Could you check a few things on this model? Use its own coordinates, in mm. A direction names the side the tool comes from. Round coordinates to 2 decimals unless told otherwise and drop trailing zeros. Write each loop counter-clockwise with the first axis right and the second up, starting at its lowest first coordinate (ties: lowest second). Pieces come first, ordered by that corner, then holes. Notation, with made-up numbers: (20.5, -37.5) -> (77.5, -37.5) arc R7 ccw to (77.5, -29.5) -> close; hole circle Ø11 at (40, -31.75). An arc over 180 degrees is marked (long way). Answer in a Markdown table with one row per item.
from build123d import *

# Parameters (mm, degrees)
SKETCH1_W           = 26
SKETCH1_H           = 10.8
BOSS_EXTRUDE1_DEPTH = 25
SKETCH2_W           = 8
SKETCH2_H           = 4
BOSS_EXTRUDE2_DEPTH = 10.25
SKETCH3_R           = 1.25
CUT_EXTRUDE1_DEPTH  = 10.25
CUT_EXTRUDE2_DEPTH  = 40.092230686
SHELL1_START        = -2.4
SHELL1_DEPTH        = 4.8
SKETCH5_W           = 4.8
SKETCH5_H           = 4.8
CUT_EXTRUDE3_DEPTH  = 10.25
SKETCH6_W           = 1
SKETCH6_H           = 1
CUT_EXTRUDE4_DEPTH  = 45.133009188
SKETCH7_W           = 1
SKETCH7_H           = 1
CUT_EXTRUDE5_DEPTH  = 10.25
FILLET1_R           = 2
FILLET2_R           = 2


# Read off the part's stored shape, not the designer's step: Shell1
with BuildPart() as part:
    # Sketch1 → Boss-Extrude1 (new body)
    with BuildSketch(Plane(origin=(0, 0, 0), x_dir=(1, 0, 0), z_dir=(0, 1, 0))):
        Rectangle(SKETCH1_W, SKETCH1_H)
    extrude(amount=BOSS_EXTRUDE1_DEPTH)

    # Sketch2 → Boss-Extrude2 (add)
    with BuildSketch(Plane(origin=(0, 25, 0), x_dir=(1, 0, 0), z_dir=(0, 1, 0))):
        with Locations((9, 0)):
            Rectangle(SKETCH2_W, SKETCH2_H)
    extrude(amount=BOSS_EXTRUDE2_DEPTH)

    # Sketch3 → Cut-Extrude1 (cut)
    with BuildSketch(Plane.XY.offset(2)):
        with Locations((9, 31.25)):
            Circle(SKETCH3_R)
        with BuildLine():
            Line((5, 31.25), (5, 37.25))
            Line((5, 37.25), (13, 37.25))
            Line((13, 37.25), (13, 31.25))
            ThreePointArc((13, 31.25), (9, 35.25), (5, 31.25))
        make_face()
    extrude(amount=-CUT_EXTRUDE1_DEPTH, mode=Mode.SUBTRACT)

    # Sketch4 → Cut-Extrude2 (cut, through all)
    with BuildSketch(Plane.XY.offset(5.4)):
        Polygon((-13, 0), (-2.8, 25), (-13, 25), align=None)
    extrude(amount=-CUT_EXTRUDE2_DEPTH, mode=Mode.SUBTRACT)

    # Shell1 outline → Shell1 (cut)
    with BuildSketch(Plane.XY.offset(SHELL1_START)):
        Polygon((10, 0), (10, 22), (-0.783911112, 22), (-9.759911112, 0), align=None)
    extrude(amount=SHELL1_DEPTH, mode=Mode.SUBTRACT)

    # Sketch5 → Cut-Extrude3 (cut)
    with BuildSketch(Plane(origin=(0, 25, 0), x_dir=(1, 0, 0), z_dir=(0, 1, 0))):
        with Locations((1.65, 0)):
            Rectangle(SKETCH5_W, SKETCH5_H)
    extrude(amount=-CUT_EXTRUDE3_DEPTH, mode=Mode.SUBTRACT)

    # Sketch6 → Cut-Extrude4 (cut, through all)
    with BuildSketch(Plane(origin=(13, 0, 0), x_dir=(0, 0, -1), z_dir=(1, 0, 0))):
        with Locations((-4.9, 0.5)):
            Rectangle(SKETCH6_W, SKETCH6_H)
        with Locations((4.9, 0.5)):
            Rectangle(SKETCH6_W, SKETCH6_H)
    extrude(amount=-CUT_EXTRUDE4_DEPTH, mode=Mode.SUBTRACT)

    # Sketch7 → Cut-Extrude5 (cut)
    with BuildSketch(Plane(origin=(0, 0, -5.4), x_dir=(-1, 0, 0), z_dir=(0, 0, -1))):
        with Locations((-12.5, 0.5)):
            Rectangle(SKETCH7_W, SKETCH7_H)
        with Locations((12.5, 0.5)):
            Rectangle(SKETCH7_W, SKETCH7_H)
    extrude(amount=-CUT_EXTRUDE5_DEPTH, mode=Mode.SUBTRACT)

    # Fillet1
    fillet1_edges = [part.edges().sort_by_distance(p)[0] for p in [
        (13, 13, 5.4),
        (-7.696, 13, 5.4),
        (-7.696, 13, -5.4),
        (13, 13, -5.4),
    ]]
    fillet(fillet1_edges, radius=FILLET1_R)

    # Fillet2
    fillet2_edges = [part.edges().sort_by_distance(p)[0] for p in [
        (12, 0.5, -4.4),
        (-12, 0.5, -4.4),
        (-12, 0.5, 4.4),
    ]]
    fillet(fillet2_edges, radius=FILLET2_R)


solid = part.part
1) For faces 5 (the face through (-0.75, 24, 0)), 6 (the face through (9, 29, 2)), 7 (the face through (2, 10, -2.4)), which set-ups out of +Z, -Z, +X, -X, +Y, -Y let a thin tool reach every point of the face, with its end or its side?
Findings:
| item | result |
|---|---|
| face 5 | +Y, -Y |
| face 6 | +Z, +X, -X, +Y |
| face 7 | -Y |
2) Please list where these lines run through material, in increasing order: line 1 (Z direction, x = 0.75, y = 19); line 2 (Y direction, x = 9, z = 0.5); line 3 (Y direction, x = 3.5, z = -2.5).
Findings:
| item | result |
|---|---|
| line 1 | z = -5.4 to -2.4, 2.4 to 5.4 |
| line 2 | y = 22 to 30, 32.5 to 35.25 |
| line 3 | y = 0 to 25 |
3) For pin 1 (0.5 mm diameter, centred on y = 0.5, z = 1, fed in from +X); pin 2 (2 mm diameter, centred on x = -3.5, y = 22, fed in from +Z); pin 3 (3 mm diameter, centred on y = 27.5, z = -1, fed in from -X), each with a flat end and sliding along its axis, tell me the tip position at first contact or that it passes through.
Findings:
| item | result |
|---|---|
| pin 1 | stops at x = 12 |
| pin 2 | stops at z = 5.33 |
| pin 3 | stops at x = 5 |
4) Thinking about a two-plate mould opening in Z: for faces 1 (the face through (-5.21, 11.15, -0.03)), 2 (the face through (3, 13, -5.4)), 3 (the face through (9.09, 35.25, 0.03)), 4 (the face through (-11.43, 0.51, 3.8)), which applies, +Z half, -Z half, draft (parallel to the pull), parting line (faces both ways), or undercut?
Findings:
| item | result |
|---|---|
| face 1 | undercut |
| face 2 | -Z half |
| face 3 | draft |
| face 4 | +Z half |
5) Imagine slicing it at A-A, the plane x = -0.25. Please give me the cut outline in (y, z).
Findings:
| item | result |
|---|---|
| outline | (0, -4.4) -> (1, -4.4) -> (1, -5.4) -> (25, -5.4) -> (25, -2.4) -> (0, -2.4) -> close; (0, 2.4) -> (25, 2.4) -> (25, 5.4) -> (1, 5.4) -> (1, 4.4) -> (0, 4.4) -> close |
6) Imagine slicing it at D-D, the plane z = 3. Please give me the cut outline in (x, y), plus the area to 3 significant figures.
Findings:
| item | result |
|---|---|
| outline | (-12.59, 1) -> (-11.91, 1) -> (-11.91, 0) -> (12, 0) -> (12, 1) -> (13, 1) -> (13, 25) -> (-2.8, 25) -> close |
| area | 521 mm^2 |
7) Imagine slicing it at B-B, the plane z = -0.5. Count the separate pieces of the cut face and the enclosed holes in it, plus the area to 3 significant figures.
Findings:
| item | result |
|---|---|
| separate pieces | 2 |
| enclosed holes | 1 |
| area | 241 mm^2 |
8) Imagine slicing it at C-C, the plane x = 9. Please give me the cut outline in (y, z), plus the area to 3 significant figures.
Findings:
| item | result |
|---|---|
| outline | (0, -4.4) -> (1, -4.4) -> (1, -5.4) -> (25, -5.4) -> (25, -2) -> (30, -2) -> (30, 2) -> (25, 2) -> (25, 5.4) -> (1, 5.4) -> (1, 4.4) -> (0, 4.4) -> (0, 2.4) -> (22, 2.4) -> (22, -2.4) -> (0, -2.4) -> close; (32.5, -2) -> (35.25, -2) -> (35.25, 2) -> (32.5, 2) -> close |
| area | 193 mm^2 |
